```python
from build123d import *

# Parameters (mm, degrees)
BOSS_EXTRUDE4_DEPTH = 304.8
SKETCH4_OUTSIDE_W   = 384.928
SKETCH4_OUTSIDE_H   = 321.428
CUT_EXTRUDE2_DEPTH  = 150
SKETCH6_R           = 3.175
CUT_EXTRUDE5_DEPTH  = 150


with BuildPart() as part:
    # Sketch3 → Boss-Extrude4 (new body)
    with BuildSketch(Plane(origin=(0, 0, 0), x_dir=(0, 0, -1), z_dir=(1, 0, 0))):
        with BuildLine():
            ThreePointArc((232.90669496, 1.961354585), (112.25669496, -30.366715482), (-8.39330504, 1.961354585))
            Line((-8.39330504, 1.961354585), (-8.39330504, -4.052041589))
            ThreePointArc((-8.39330504, -4.052041589), (112.25669496, -36.380111656), (232.90669496, -4.052041589))
            Line((232.90669496, -4.052041589), (232.90669496, 1.961354585))
        make_face()
    extrude(amount=BOSS_EXTRUDE4_DEPTH)

    # Sketch4 outside → Cut-Extrude2 (cut)
    with BuildSketch(Plane(origin=(0, 1.961354585, 0), x_dir=(1, 0, 0), z_dir=(0, 1, 0))):
        with Locations((152.4, 112.257)):
            Rectangle(SKETCH4_OUTSIDE_W, SKETCH4_OUTSIDE_H)
        Polygon((105.356331211, 184.098739751), (33.514261355, 112.256736733), (105.356310324, 40.414687765), (123.316822566, 58.375200007), (69.435327613, 112.25669496), (123.316851808, 166.138219154), align=None, mode=Mode.SUBTRACT)
    extrude(amount=-CUT_EXTRUDE2_DEPTH, mode=Mode.SUBTRACT)

    # Sketch6 → Cut-Extrude5 (cut)
    with BuildSketch(Plane(origin=(0, 1.961354585, 0), x_dir=(1, 0, 0), z_dir=(0, 1, 0))):
        with Locations(Location((97.916821174, 167.678955491, 0), (0, 0, 270))):
            Circle(SKETCH6_R)
        with Locations(Location((106.897078687, 158.698700762, 0), (0, 0, 270))):
            Circle(SKETCH6_R)
        with Locations(Location((60.455057568, 130.217250368, 0), (0, 0, 270))):
            Circle(SKETCH6_R)
        with Locations(Location((69.435303942, 121.2369845, 0), (0, 0, 270))):
            Circle(SKETCH6_R)
        with Locations(Location((60.455015794, 94.296160438, 0), (0, 0, 270))):
            Circle(SKETCH6_R)
        with Locations(Location((69.435283055, 103.27640542, 0), (0, 0, 270))):
            Circle(SKETCH6_R)
        with Locations(Location((106.89697067, 65.814602027, 0), (0, 0, 270))):
            Circle(SKETCH6_R)
        with Locations(Location((97.916692269, 56.834368185, 0), (0, 0, 270))):
            Circle(SKETCH6_R)
    extrude(amount=-CUT_EXTRUDE5_DEPTH, mode=Mode.SUBTRACT)


solid = part.part
```
Geometry: final body of the model. Coordinates: model frame, mm. A direction names the side the tool comes from. Coordinates: 2 decimals unless noted, no trailing zeros. Order: outer loops, then holes, each group sorted by start corner. A loop starts at its lowest first (then second) coordinate and runs counter-clockwise, first axis right, second up. Notation, with made-up numbers: M 79.5,18.25 L 124.5,18.25 A15 cw 124.5,38.25 Z; hole C -2.5,59 d3. An arc over 180 degrees is marked long. Answer in a Markdown table with one row per item. Add a question column.
Q1. Section query C-C on z = -51.5. Return the cut outline in (x, y).
Q2. Reachability of faces 4 (the flat face through (96.75, -31.59, -84.94)), 5 (the cylindrical face through (62.6, -32.63, -132.56)) from +Z, -Z, +X, -X, +Y, -Y: full face, straight path, thin tool, end or side. Return the list, or none.
Q3. Contact query for flat-ended pins moving along their axis: P1, Ø12, axis at x = 89, z = -63.5, coming from the +Y side; P2, Ø8.5, axis at x = 106.9, z = -65.81, coming from the -Y side; P3, Ø5, axis at x = 69.44, z = -103.28, coming from the +Y side; P4, Ø10, axis at x = 69.44, z = -121.24, coming from the +Y side. Output: stop coordinate, or through.
Q4. Mould query, pull axis X, two halves, no side actions, for faces 1 (the flat face through (114.462, -24.78, -174.993)), 2 (the cylindrical face through (100.594, -26.854, -55.128)), 3 (the flat face through (69.27, -29.12, -76.5)). Classes: released by +X, released by -X, zero draft, split by the parting line, or undercut.
Q5. Section query D-D on x = 53.5. Return the cut outline in (y, z).
Q6. Line query: L1, parallel to X at y = -25, z = -58; L2, parallel to Z at x = 73, y = -33; L3, parallel to Z at x = 64, y = -31. Output: solid intervals per line, ascending.
Q7. Section query A-A on x = 80.5. Return the cut outline in (y, z).
Completed:
| question | item | result |
|---|---|---|
| 1 | outline | M 94.27,-28.61 L 116.44,-28.61 L 116.44,-22.59 L 94.27,-22.59 Z |
| 2 | face 4 | +X, +Y, -Y |
| 2 | face 5 | +Y, -Y |
| 3 | P1 | stops at y = -24.07 |
| 3 | P2 | stops at y = -32.66 |
| 3 | P3 | passes through |
| 3 | P4 | stops at y = -29.96 |
| 4 | face 1 | released by +X |
| 4 | face 2 | undercut |
| 4 | face 3 | released by -X |
| 5 | outline | M -35.55,-132.24 L -29.54,-132.24 A241.3 cw -29.54,-92.27 L -35.55,-92.27 A241.3 ccw Z |
| 6 | L1 | x = 87.77 to 94.96, 100.87 to 122.94 |
| 6 | L2 | z = -151.74 to -115.82, -108.69 to -72.77 |
| 6 | L3 | z = -142.74 to -81.77 |
| 7 | outline | M -36.13,-123.32 A241.3 ccw -31.76,-159.24 L -25.75,-159.24 A241.3 cw -30.11,-123.32 Z; M -36.13,-101.19 L -30.11,-101.19 A241.3 cw -25.75,-65.27 L -31.76,-65.27 A241.3 ccw Z |
